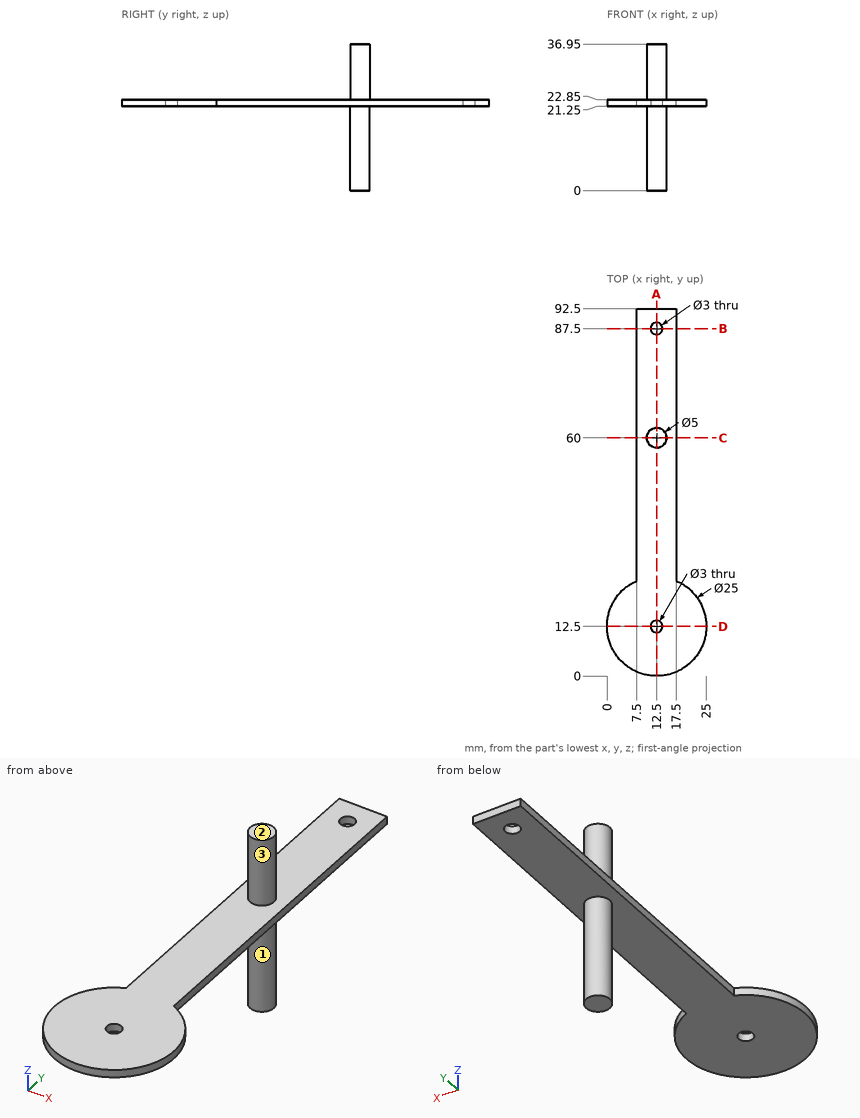
Check sheet for the drawn part. Datum: minimum x, y, z corner. Units: mm. A direction names the side the tool comes from. Round coordinates to 2 decimals unless told otherwise and drop trailing zeros. Order: outer loops, then holes, each group sorted by start corner. A loop starts at its lowest first (then second) coordinate and runs counter-clockwise, first axis right, second up.
1) Section check B-B (y = 87.5). Record the boundary of the cut face in (x, z).
2) Go/stop test with flat-tipped pins: pin 1 Ø2 at (x, y) = (13, 48.5) entering from -Z; pin 2 Ø6 at (x, y) = (6, 74) entering from +Z; pin 3 Ø0.5 at (y, z) = (65, 22) entering from -X. Record where each tip stops, or that it passes through.
3) Section check C-C (y = 60). Record the boundary of the cut face in (x, z).
4) Scan lines: line 1 (Y direction, x = 12.5, z = 22.1); line 2 (X direction, y = 87.5, z = 22.1); line 3 (Z direction, x = 12.5, y = 27.5). Record each from-to range of solid material in increasing order.
5) Tool access check on the marked faces 1, 2 and 3. Record the directions out of +Z, -Z, +X, -X, +Y, -Y that give a thin tool (end or side, any length) a straight path to the whole face; none if there is none.
6) Section check D-D (y = 12.5). Record the boundary of the cut face in (x, z).
7) Section check A-A (x = 12.5). Record the boundary of the cut face in (y, z).
Result:
1. outline: (7.5, 21.25) - (11, 21.25) - (11, 22.85) - (7.5, 22.85) - close; (14, 21.25) - (17.5, 21.25) - (17.5, 22.85) - (14, 22.85) - close
2. pin 1: stops at z = 21.25
2. pin 2: stops at z = 22.85
2. pin 3: stops at x = 7.5
3. outline: (7.5, 21.25) - (10, 21.25) - (10, 0) - (15, 0) - (15, 21.25) - (17.5, 21.25) - (17.5, 22.85) - (15, 22.85) - (15, 36.95) - (10, 36.95) - (10, 22.85) - (7.5, 22.85) - close
4. line 1: y = 0 to 11, 14 to 86, 89 to 92.5
4. line 2: x = 7.5 to 11, 14 to 17.5
4. line 3: z = 21.25 to 22.85
5. face 1: -Z
5. face 2: +Z, +X, -X, +Y, -Y
5. face 3: +Z
6. outline: (0, 21.25) - (11, 21.25) - (11, 22.85) - (0, 22.85) - close; (14, 21.25) - (25, 21.25) - (25, 22.85) - (14, 22.85) - close
7. outline: (0, 21.25) - (11, 21.25) - (11, 22.85) - (0, 22.85) - close; (14, 21.25) - (57.5, 21.25) - (57.5, 0) - (62.5, 0) - (62.5, 21.25) - (86, 21.25) - (86, 22.85) - (62.5, 22.85) - (62.5, 36.95) - (57.5, 36.95) - (57.5, 22.85) - (14, 22.85) - close; (89, 21.25) - (92.5, 21.25) - (92.5, 22.85) - (89, 22.85) - close
